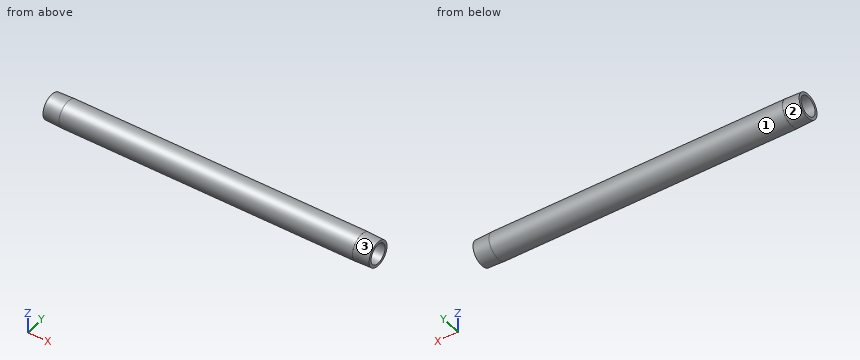
Autodesk Inventor part; units mm, degrees
ref_plane "YZ Plane" through (0, 0, 0) normal (1, 0, 0) x (0, 1, 0)
ref_plane "XZ Plane" through (0, 0, 0) normal (0, 1, 0) x (-1, 0, 0)
ref_plane "XY Plane" through (0, 0, 0) normal (0, 0, 1) x (1, 0, 0)
sketch "Sketch1" plane through (0, 0, 0) normal (0, 1, 0) x (-1, 0, 0)
  line L0 (-264.16, 0) -> (0, 0)
  line L1 (0, 0) -> (0, 8.05) construction
  line L2 (0, 8.05) -> (0, 10.2212)
  line L3 (0, 10.2212) -> (-13.2, 10.6337)
  line L4 (-13.2, 10.6337) -> (-13.2281, 10.65)
  line L5 (-13.2281, 10.65) -> (-250.9319, 10.65)
  line L6 (0, 8.05) -> (-264.16, 8.05)
  line L7 (-132.08, 0) -> (-132.08, 10.65) construction
  line L8 (-264.16, 0) -> (-264.16, 8.05) construction
  line L9 (-264.16, 8.05) -> (-264.16, 10.2212)
  line L10 (-264.16, 10.2212) -> (-250.96, 10.6337)
  line L11 (-250.96, 10.6337) -> (-250.9319, 10.65)
  line L12 (-8.2, 10.4775) -> (-8.2, 0) construction
  line L13 (-13.2, 10.6337) -> (-13.2, 0) construction
  line L14 (-250.96, 10.6337) -> (-250.96, 0) construction
  dimension "d0" = 8.2
  dimension "d1" = 13.2
  dimension "d2" = 1.79
  dimension "d3" = 20.955
  dimension "d4" = 21.3
  dimension "d5" = 2.6
  dimension "d6" = 264.16
  dimension "d7" = 30
revolve "Revolution1" add sketch "Sketch1" angle 360 about axis through (264.16, 0, 0) along (-1, 0, 0)
thread "Thread1"
thread "Thread2"
equation "\"d0\" = a"
equation "\"d1\" = LT"
equation "\"d3\" = MjD"
equation "\"d4\" = OD"
equation "\"d5\" = T"
equation "\"d6\" = L"
equation "\"OD\" = 21.3"
equation "\"T\" = 2.6"
equation "\"L\" = PL"
equation "\"LT\" = 13.2"
equation "\"ID\" = 16.1"
equation "\"PL\" = 264.16"
equation "\"MjD\" = 20.955"
equation "\"a\" = 8.2"
equation "\"Size_Designation\" = 1.2345"
equation "\"PLmin\" = 2 * LT + T"
properties material "Stainless Steel"
Part model, mm, in its own coordinate system. Face numbers are marked on the shaded views. A direction names the side the tool comes from. Give positions to 0.01 mm unless a question says otherwise; leave off trailing zeros. Write each loop counter-clockwise with the first axis right and the second up, starting at its lowest first coordinate (ties: lowest second). Pieces come first, ordered by that corner, then holes.
1) Cut at C-C on x = 49. Write the cut outline in (y, z), then the cut area to 3 significant figures.
Resolved:
outline: circle Ø21.3 at (0, 0); hole circle Ø16.1 at (0, 0)
area: 153 mm2
2) Which spindle directions (+Z, -Z, +X, -X, +Y, -Y) get a long thin tool onto all of the face, cutting with end or side? Do the marked faces 1, 2 and 3. Say none if no direction does.
Resolved:
face 1: +X, -X
face 2: -X
face 3: +X
3) Pin check, flat tips, straight feed: pin 1 (5 mm diameter, centred on x = 233.5, y = -5.5, fed in from +Z); pin 2 (10 mm diameter, centred on x = 59, z = 5, fed in from -Y); pin 3 (8 mm diameter, centred on x = 109, y = -8, fed in from +Z); pin 4 (1 mm diameter, centred on x = 71, y = -4, fed in from +Z). Stop position of each tip, or through.
Resolved:
pin 1: stops at z = 10.22
pin 2: stops at y = -10.65
pin 3: stops at z = 9.87
pin 4: stops at z = 10.06
4) Probe L1, parallel to Y at x = 246, z = 0.5; L2, parallel to Y at x = 97, z = -3.25; L3, parallel to Z at x = 32.5, y = -6.75. List the from-to ranges inside material, lowest first.
Resolved:
L1: y = -10.64 to -8.03, 8.03 to 10.64
L2: y = -10.14 to -7.36, 7.36 to 10.14
L3: z = -8.24 to -4.39, 4.39 to 8.24
